Design review of the part built by this model. Coordinates are the model's own, in mm. Face numbers are marked on the shaded views. Give positions to 0.01 mm unless a question says otherwise; leave off trailing zeros. Write each loop counter-clockwise with the first axis right and the second up, starting at its lowest first coordinate (ties: lowest second). Pieces come first, ordered by that corner, then holes. Notation, with made-up numbers: M 74,-19.5 L 86,-19.5 A19 cw 86,-1.5 Z; hole C 45,59 d10. An arc over 180 degrees is marked long. Write each question's results on one line, items separated by ' | '. Start each with the question number.
from build123d import *

# Parameters (mm, degrees)
SKETCH_1_W             = 32
SKETCH_1_H             = 5
EXTRUDE_1_DEPTH        = 8.75
CUT_EXTRUDE_1_DEPTH    = 24.843238035
PATTERN_LINEAR_1_COUNT = 11
PATTERN_LINEAR_1_PITCH = 3
SKETCH_3_W             = 1.5
SKETCH_3_H             = 1.22
SKETCH_3_W_2           = 0.5
CUT_EXTRUDE_2_DEPTH    = 24.843238035
SKETCH_4_R             = 1.6
CUT_EXTRUDE_3_DEPTH    = 19.909323097
CHAMFER_1_SIZE         = 1.5
FILLET_1_R             = 3.5


with BuildPart() as part:
    # 草图1 → 凸台-拉伸1 (new, symmetric)
    with BuildSketch(Plane.XY):
        Rectangle(SKETCH_1_W, SKETCH_1_H)
    extrude(amount=EXTRUDE_1_DEPTH, both=True)

    # 草图2 → 切除-拉伸1 (cut, through all)
    with BuildSketch(Plane.XY.offset(8.75)):
        with BuildLine():
            Line((-16, -2.5), (-15.63, -2.5))
            ThreePointArc((-15.63, -2.5), (-15.460294373, -2.429705627), (-15.39, -2.26))
            Line((-15.39, -2.26), (-15.39, -2.17))
            ThreePointArc((-15.39, -2.17), (-14.5, -1.28), (-13.61, -2.17))
            Line((-13.61, -2.17), (-13.61, -2.26))
            ThreePointArc((-13.61, -2.26), (-13.539705627, -2.429705627), (-13.37, -2.5))
            Line((-13.37, -2.5), (-13, -2.5))
            Line((-13, -2.5), (-13, -3.5))
            Line((-13, -3.5), (-16, -3.5))
            Line((-16, -3.5), (-16, -2.5))
        make_face()
    cut_extrude_1 = extrude(amount=-CUT_EXTRUDE_1_DEPTH, mode=Mode.SUBTRACT)

    # 阵列(线性)1: 切除-拉伸1 ×11
    with Locations(*[(i * PATTERN_LINEAR_1_PITCH, 0, 0) for i in range(1, PATTERN_LINEAR_1_COUNT)]):
        add(cut_extrude_1, mode=Mode.SUBTRACT)

    # 草图3 → 切除-拉伸2 (cut, through all)
    with BuildSketch(Plane.XY.offset(8.75)):
        with Locations((-15.25, -1.89)):
            Rectangle(SKETCH_3_W, SKETCH_3_H)
        with Locations((15.75, -1.89)):
            Rectangle(SKETCH_3_W_2, SKETCH_3_H)
    extrude(amount=-CUT_EXTRUDE_2_DEPTH, mode=Mode.SUBTRACT)

    # 草图4 → 切除-拉伸3 (cut, through all)
    with BuildSketch(Plane(origin=(0, 2.5, 0), x_dir=(1, 0, 0), z_dir=(0, 1, 0))):
        with Locations(Location((-12.5, -5.25, 0), (0, 0, 180))):
            Circle(SKETCH_4_R)
        with Locations(Location((12.5, -5.25, 0), (0, 0, 180))):
            Circle(SKETCH_4_R)
    extrude(amount=-CUT_EXTRUDE_3_DEPTH, mode=Mode.SUBTRACT)

    # 倒角1
    chamfer_1_edges = [part.edges().sort_by_distance(p)[0] for p in [
        (-10.9, 2.5, 5.25),
        (14.1, 2.5, 5.25),
    ]]
    chamfer(chamfer_1_edges, length=CHAMFER_1_SIZE)

    # 圆角1
    fillet_1_edges = [part.edges().sort_by_distance(p)[0] for p in [
        (-16, 0.61, 8.75),
        (16, 0.61, 8.75),
    ]]
    fillet(fillet_1_edges, radius=FILLET_1_R)


solid = part.part
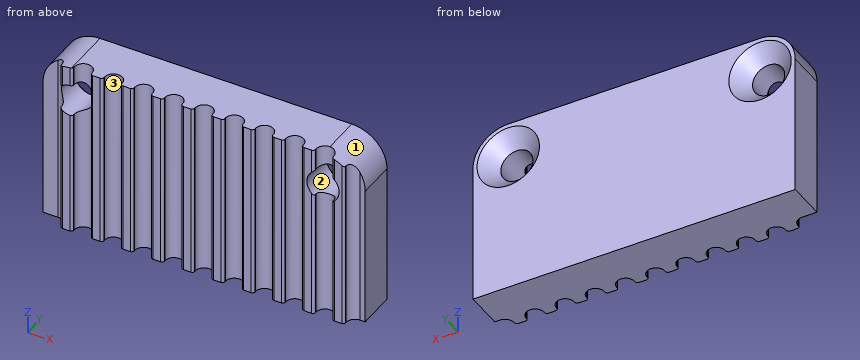
Q1. For pin 1 Ø1.9 at (x, z) = (-12.5, 5.25) entering from +Y, flat-tipped, find the tip position at first contact; note if it passes through.
Q2. Wall thickness on line 1 along X through (y, z) = (-0.8, 5.25); line 2 along Z through (x, y) = (-12.5, -1.75): over which ranges is each line inside the solid? List them lowest first. Write a range as from..to.
Q3. We need section C-C on x = -8.5. Write out the cut boundary in (y, z), and give its area (4 significant figures).
Q4. We need section B-B on y = 1.8. Write out the cut boundary in (x, z), and give its area (3 significant figures).
Q5. The part is to be moulded in two halves that separate along Z. For the marked faces 1, 2 and 3, say which applies: pulls with the +Z half, pulls with the -Z half, needs draft (parallel to the pull), parting line crosses it, or undercut.
Q6. We need section A-A on y = -0.65. Write out the cut boundary in (x, z), and give its area (3 significant figures).
Answer sheet:
1) pin 1: through
2) line 1: -16..-14.1, -10.9..10.9, 14.1..16 | line 2: -8.75..3.65, 6.85..8.75
3) outline: M -1.28,-8.75 L 2.5,-8.75 L 2.5,8.75 L -1.28,8.75 Z | area: 66.15 mm^2
4) outline: M -16,-8.75 L 16,-8.75 L 16,5.25 A3.5 ccw 12.5,8.75 L -12.5,8.75 A3.5 ccw -16,5.25 Z; hole C -12.5,5.25 d4.8; hole C 12.5,5.25 d4.8 | area: 519 mm^2
5) face 1: pulls with the +Z half | face 2: undercut | face 3: needs draft
6) outline: M -16,-8.75 L 16,-8.75 L 16,5.25 A3.5 ccw 12.5,8.75 L -12.5,8.75 A3.5 ccw -16,5.25 Z; hole C -12.5,5.25 d3.2; hole C 12.5,5.25 d3.2 | area: 539 mm^2
